from build123d import *

# Parameters (mm, degrees)
F1_DEPTH = 85
F2_START = 22.5
F2_DEPTH = 40
F4_D     = 10
F4_DEPTH = 12
F4_START = 1.4311325
F4_TIP   = 3.0043030951


# Not quite as in the source:
# - a feature names something its author has since deleted; it is built from what else it names


with BuildPart() as f1:
    # F0 (on Front) → F1 (new body)
    with BuildSketch(Plane.XZ):
        with BuildLine():
            Line((-50, -4), (50, -4))
            Line((50, -4), (50, 4))
            Line((50, 4), (46, 4))
            Line((46, 4), (-45, 4))
            ThreePointArc((-45, 4), (-48.5355339059, 2.5355339059), (-50, -1))
            Line((-50, -1), (-50, -4))
        make_face()
        with BuildLine():
            Line((-6.7640438608, 111.7814914912), (-4.3106391095, 114.9407327175))
            ThreePointArc((-4.3106391095, 114.9407327175), (-7.8808210545, 115.6224300093), (-10.5289002901, 113.1327339074))
            Line((-10.5289002901, 113.1327339074), (-6.7640438608, 111.7814914912))
        make_face()
        with BuildLine():
            Line((46, 4), (50, 4))
            ThreePointArc((50, 4), (35.6938059368, 65.7606098099), (-4.3106391095, 114.9407327175))
            Line((-4.3106391095, 114.9407327175), (-6.7640438608, 111.7814914912))
            ThreePointArc((-6.7640438608, 111.7814914912), (32.1012011015, 64.0018629557), (46, 4))
        make_face()
        Polygon((-42.2341572851, 12.9540102238), (-6.7640438608, 111.7814914912), (-10.5289002901, 113.1327339074), (-44.6477712982, 18.0701090692), (-45.9990137144, 14.3052526399), align=None)
        Polygon((-45.9990137144, 14.3052526399), (-44.6477712982, 18.0701090692), (-55.9423405859, 22.1238363177), (-57.2935830021, 18.3589798884), align=None)
    extrude(amount=F1_DEPTH)

    # F0 (on Front) → F2 (cut)
    with BuildSketch(Plane.XZ.offset(F2_START)):
        Polygon((-45.9990137144, 14.3052526399), (-44.6477712982, 18.0701090692), (-55.9423405859, 22.1238363177), (-57.2935830021, 18.3589798884), align=None)
    extrude(amount=F2_DEPTH, mode=Mode.SUBTRACT)

    # F4
    # its depths count from where the whole tool has entered the part; down to there all is cleared
    with Locations(Plane.YZ.offset(50).offset(-F4_START)):
        with Locations((-42.5, 19)):
            Hole(F4_D / 2, depth=F4_DEPTH)
            with Locations((0, 0, -(F4_DEPTH + F4_TIP / 2))):  # 118° drill point
                Cone(0, F4_D / 2, F4_TIP, mode=Mode.SUBTRACT)


solid = f1.part
Source: CAD feature listing. Evaluate the final solid. Frame: model axes, mm. A direction names the side the tool comes from. Coordinates: 2 decimals unless noted, no trailing zeros. Loops run counter-clockwise (first coordinate to the right, second up) from the corner with the lowest first, then second, coordinate; pieces in that order, holes last. Notation, with made-up numbers: (-7.5, 55) - (22.5, 55) arc R24 cw to (22.5, 77) - close; hole circle Ø3 at (21, 17.5). An arc over 180 degrees is marked (long way). Return JSON: item names as keys, results as strings.
Q1. Mould query, pull axis Y, two halves, no side actions, for faces 5 (the cylindrical face through (47.049, -38.815, 22.379)), 6 (the flat face through (-51, -22.5, 18)), 7 (the flat face through (-1, -42, -4)), 8 (the flat face through (-4, 0, 3)). Classes: released by +Y, released by -Y, zero draft, split by the parting line, or undercut.
Results:
{"face 5": "undercut", "face 6": "undercut", "face 7": "zero draft", "face 8": "released by +Y"}
Q2. Access query for faces 1 (the flat face through (-50, -42, -2)), 2 (the flat face through (1, -42, 4)), 3 (the flat face through (-51, -62.5, 18)), 4 (the flat face through (-24.747, -41.905, 61.676)). Directions: +Z, -Z, +X, -X, +Y, -Y. A direction counts if a zero-diameter tool reaches every point of the face in a straight line with its end or side. Return the directions, or none.
Results:
{"face 1": "-Z, -X, +Y, -Y", "face 2": "-X, +Y, -Y", "face 3": "+Z, -X", "face 4": "+Y, -Y"}
Q3. Material intervals for line 1 along Y through (x, z) = (46.65, 19); line 2 along X through (y, z) = (-8.5, 109.5); line 3 along X through (y, z) = (-38.5, 47), sorted ascending.
Results:
{"line 1": "-85 to -47.5, -37.5 to 0", "line 2": "-11.83 to -7.58, -3.91 to 2.27", "line 3": "-34.26 to -30.01, 39.05 to 43.26"}
Q4. Section D-D, the plane x = 36.5. Return loops of the section in (y, z).
Results:
{"outline": "(-85, -4) - (0, -4) - (0, 4) - (-85, 4) - close; (-85, 54.03) - (0, 54.03) - (0, 64.09) - (-85, 64.09) - close"}
Q5. Section B-B, the plane y = -79. Return loops of the section in (x, z).
Results:
{"outline": "(-57.29, 18.36) - (-42.23, 12.95) - (-6.76, 111.78) arc R136.47 cw to (46, 4) - (-45, 4) arc R5 ccw to (-50, -1) - (-50, -4) - (50, -4) - (50, 4) arc R140.47 ccw to (-4.31, 114.94) arc R4 ccw to (-10.53, 113.13) - (-44.65, 18.07) - (-55.94, 22.12) - close"}
Q6. Section A-A, the plane z = 84.5. Return loops of the section in (x, y).
Results:
{"outline": "(-20.81, -85) - (-16.56, -85) - (-16.56, 0) - (-20.81, 0) - close; (19.73, -85) - (24.64, -85) - (24.64, 0) - (19.73, 0) - close"}
Q7. Section C-C, the plane y = -41. Return loops of the section in (x, z), plus the area to 3 significant figures.
Results:
{"outline": "(-50, -4) - (50, -4) - (50, 4) arc R140.47 ccw to (49.63, 14.23) - (45.62, 14.23) arc R136.47 cw to (46, 4) - (-45, 4) arc R5 ccw to (-50, -1) - close; (-46, 14.31) - (-42.23, 12.95) - (-6.76, 111.78) arc R136.47 cw to (44.56, 23.77) - (48.6, 23.77) arc R140.47 ccw to (-4.31, 114.94) arc R4 ccw to (-10.53, 113.13) - close", "area": "1,700 mm2"}
Q8. Contact query for flat-ended pins moving along their axis: P1, Ø5, axis at x = 16.5, y = -56, coming from the +Z side; P2, Ø6, axis at y = -42.5, z = 19, coming from the +X side; P3, Ø3, axis at x = 21.5, y = -68, coming from the +Z side. Output: stop coordinate, or through.
Results:
{"P1": "z = 97.9", "P2": "x = -38.99", "P3": "z = 90.76"}
